```python
from build123d import *

# Parameters (mm, degrees)
F0_W     = 152.4
F0_H     = 127
F1_DEPTH = 127
F3_DEPTH = 76.2
F4_W     = 50.8
F4_H     = 41.993012
F5_DEPTH = 50.8
F7_SIZE  = 25.4
F6_R     = 21.59
F8_DEPTH = 50.801
F9_R     = 38.1


with BuildPart() as f1:
    # F0 (on Top) → F1 (new body)
    with BuildSketch(Plane.XY):
        with Locations((1.093576, 7.667228)):
            Rectangle(F0_W, F0_H)
    extrude(amount=F1_DEPTH)

    # F2 (on face) → F3 (cut)
    with BuildSketch(Plane.XY.offset(127)):
        Polygon((26.493576, 29.174216), (-24.306424, 29.174216), (-24.306424, -55.832772), (77.293576, -55.832772), (77.293576, 29.174216), align=None)
    extrude(amount=-F3_DEPTH, mode=Mode.SUBTRACT)

    # F4 (on face) → F5 (cut)
    with BuildSketch(Plane.XY.offset(127)):
        with Locations((1.093576, 50.170722)):
            Rectangle(F4_W, F4_H)
    extrude(amount=-F5_DEPTH, mode=Mode.SUBTRACT)

    # F7
    f7_edges = [f1.edges().sort_by_distance(p)[0] for p in [
        (77.293576, 50.170722, 127),
    ]]
    chamfer(f7_edges, length=F7_SIZE)

    # F6 (on face) → F8 (cut, through all)
    with BuildSketch(Plane.XY.offset(50.8)):
        with Locations((23.953576, -12.652772)):
            Circle(F6_R)
    extrude(amount=-F8_DEPTH, mode=Mode.SUBTRACT)

    # F9
    f9_edges = [f1.edges().sort_by_distance(p)[0] for p in [
        (-49.706424, -55.832772, 127),
    ]]
    fillet(f9_edges, radius=F9_R)


solid = f1.part
```
The model under review builds one solid part; all positions refer to its coordinate system, in mm. A direction names the side the tool comes from. Round coordinates to 2 decimals unless told otherwise and drop trailing zeros. Order: outer loops, then holes, each group sorted by start corner. A loop starts at its lowest first (then second) coordinate and runs counter-clockwise, first axis right, second up. Notation, with made-up numbers: (-23, 35) -> (36, 35) arc R19 cw to (36, 55) -> close; hole circle Ø3 at (-35.5, -18.75). An arc over 180 degrees is marked (long way). Use a Markdown table: item, result.
Q1. We need section A-A on z = 98.5. Write out the cut boundary in (x, y), then the cut area to 3 significant figures.
Values:
| item | result |
|---|---|
| outline | (-75.11, -54.6) -> (-24.31, -54.6) -> (-24.31, 71.17) -> (-75.11, 71.17) -> close; (26.49, 29.17) -> (77.29, 29.17) -> (77.29, 71.17) -> (26.49, 71.17) -> close |
| area | 8,520 mm^2 |
Q2. Clearance check with flat-ended pins moving along their axes: P1, Ø21, axis at x = -4.5, y = 51.5, coming from the +Z side; P2, Ø23, axis at y = 3.5, z = 100, coming from the +X side; P3, Ø10, axis at x = 33, z = 60, coming from the -Y side; P4, Ø6, axis at x = 12, y = -23, coming from the -Z side. State where each tip first meets the part, or that it passes through.
Values:
| item | result |
|---|---|
| P1 | stops at z = 76.2 |
| P2 | stops at x = -24.31 |
| P3 | stops at y = 29.17 |
| P4 | passes through |
Q3. Mouldability with a two-part tool opening along Y and no side actions: class faces 5 (the flat face through (38, 29.174, 81)), 6 (the cylindrical face through (6.82, -25.79, 25.76)), 7 (the flat face through (-75.106, 7, 63)) as +Y half, -Y half, draft (parallel to the pull), parting line (faces both ways), or undercut.
Values:
| item | result |
|---|---|
| face 5 | -Y half |
| face 6 | undercut |
| face 7 | draft |
Q4. We need section C-C on x = 9.5. Write out the cut boundary in (y, z), then the cut area to 3 significant figures.
Values:
| item | result |
|---|---|
| outline | (-55.83, 0) -> (-28.69, 0) -> (-28.69, 50.8) -> (-55.83, 50.8) -> close; (3.39, 0) -> (71.17, 0) -> (71.17, 76.2) -> (29.17, 76.2) -> (29.17, 50.8) -> (3.39, 50.8) -> close |
| area | 5,890 mm^2 |
Q5. Tool access review of faces 1 (the flat face through (1, 50, 76.2)), 2 (the flat face through (-24.306, 9, 89)), 3 (the flat face through (37, 6, 50.8)), 4 (the flat face through (0, 71.167, 48)): name each direction out of +Z, -Z, +X, -X, +Y, -Y from which nothing blocks a thin tool from reaching the whole face with its end or side.
Values:
| item | result |
|---|---|
| face 1 | +Z, +Y, -Y |
| face 2 | +Z, -Y |
| face 3 | +Z, +X, -Y |
| face 4 | +Z, -Z, +X, -X, +Y |
Q6. We need section D-D on z = 72.5. Write out the cut boundary in (x, y).
Values:
| item | result |
|---|---|
| outline | (-75.11, -55.83) -> (-24.31, -55.83) -> (-24.31, 29.17) -> (77.29, 29.17) -> (77.29, 71.17) -> (-75.11, 71.17) -> close |
Q7. We need section B-B on y = 43. Write out the cut boundary in (x, z).
Values:
| item | result |
|---|---|
| outline | (-75.11, 0) -> (77.29, 0) -> (77.29, 101.6) -> (51.89, 127) -> (26.49, 127) -> (26.49, 76.2) -> (-24.31, 76.2) -> (-24.31, 127) -> (-75.11, 127) -> close |
Q8. For line 1 (X direction, y = -16, z = 52.5); line 2 (Z direction, x = -21.5, y = -1); line 3 (Y direction, x = 23, z = 76), list the stretches that pass through material, from the lowest coordinate up.
Values:
| item | result |
|---|---|
| line 1 | x = -75.11 to -24.31 |
| line 2 | z = 0 to 50.8 |
| line 3 | y = 29.17 to 71.17 |
